```python
from build123d import *

# Parameters (mm, degrees)
SKETCH_1_W           = 185
SKETCH_1_H           = 55
EXTRUDE_1_DEPTH      = 25
SHELL_1_T            = -2
SKETCH_8_R           = 2.15
EXTRUDE_3_DEPTH      = 4
SKETCH_2_W           = 10
SKETCH_2_H           = 4
SKETCH_2_W_2         = 5
SKETCH_2_H_2         = 5
SKETCH_2_R           = 1.4
SKETCH_2_W_3         = 170
EXTRUDE_4_DEPTH      = 6
SKETCH_2_6_R         = 2.8
SKETCH_2_6_R_2       = 1.4
EXTRUDE_6_DEPTH      = 23
SKETCH_9_W           = 30
SKETCH_9_H           = 11
CUT_EXTRUDE_7_DEPTH  = 5
SKETCH_10_W          = 177
SKETCH_10_H          = 7.5
CUT_EXTRUDE_8_DEPTH  = 5
SKETCH_11_W          = 21.2
SKETCH_11_H          = 7.5
CUT_EXTRUDE_9_DEPTH  = 5
SKETCH_12_W          = 174
SKETCH_12_H          = 7.5
CUT_EXTRUDE_10_DEPTH = 5


with BuildPart() as part:
    # Sketch 1 → Extrude 1 (new body)
    with BuildSketch(Plane(origin=(0, 0, 0), x_dir=(1, 0, 0), z_dir=(0, 1, 0))):
        Rectangle(SKETCH_1_W, SKETCH_1_H)
    extrude(amount=EXTRUDE_1_DEPTH)

    # Shell 1
    shell_1_openings = [part.faces().sort_by_distance(p)[0] for p in [
        (0, 25, 0),
    ]]
    offset(amount=SHELL_1_T, openings=shell_1_openings, kind=Kind.INTERSECTION)

    # Sketch 8 → Extrude 3 (add)
    with BuildSketch(Plane.XZ):
        with BuildLine():
            Line((-97.5, 5), (-96, 5))
            Line((-96, 5), (-96, 27.5))
            Line((-96, 27.5), (-92.5, 27.5))
            Line((-92.5, 27.5), (-92.5, -27.5))
            Line((-92.5, -27.5), (-96, -27.5))
            Line((-96, -27.5), (-96, -5))
            Line((-96, -5), (-97.5, -5))
            ThreePointArc((-97.5, -5), (-102.5, 0), (-97.5, 5))
        make_face()
        with Locations((-97.5, 0)):
            Circle(SKETCH_8_R, mode=Mode.SUBTRACT)
        with BuildLine():
            Line((97.5, -5), (96, -5))
            Line((96, -5), (96, -27.5))
            Line((96, -27.5), (92.5, -27.5))
            Line((92.5, -27.5), (92.5, -5))
            Line((92.5, -5), (92.5, 5))
            Line((92.5, 5), (92.5, 27.5))
            Line((92.5, 27.5), (96, 27.5))
            Line((96, 27.5), (96, 5))
            Line((96, 5), (97.5, 5))
            ThreePointArc((97.5, 5), (102.5, 0), (97.5, -5))
        make_face()
        with Locations((97.5, 0)):
            Circle(SKETCH_8_R, mode=Mode.SUBTRACT)
    extrude(amount=-EXTRUDE_3_DEPTH)

    # Sketch 2 → Extrude 4 (add)
    with BuildSketch(Plane(origin=(0, 2, 0), x_dir=(1, 0, 0), z_dir=(0, 1, 0))):
        with Locations((-85.5, 23.4)):
            Rectangle(SKETCH_2_W, SKETCH_2_H)
        with Locations((-74.6, 12.65)):
            Rectangle(SKETCH_2_W_2, SKETCH_2_H_2)
        with Locations((-74.6, 12.65)):
            Circle(SKETCH_2_R, mode=Mode.SUBTRACT)
        with Locations((74.6, -12.65)):
            Rectangle(SKETCH_2_W_2, SKETCH_2_H_2)
        with Locations((74.6, -12.65)):
            Circle(SKETCH_2_R, mode=Mode.SUBTRACT)
        with Locations((74.6, 12.65)):
            Rectangle(SKETCH_2_W_2, SKETCH_2_H_2)
        with Locations((74.6, 12.65)):
            Circle(SKETCH_2_R, mode=Mode.SUBTRACT)
        with Locations((0, -12.65)):
            Rectangle(SKETCH_2_W_2, SKETCH_2_H_2)
        with Locations((0, -12.65)):
            Circle(SKETCH_2_R, mode=Mode.SUBTRACT)
        with Locations((0, 12.65)):
            Rectangle(SKETCH_2_W_2, SKETCH_2_H_2)
        with Locations((0, 12.65)):
            Circle(SKETCH_2_R, mode=Mode.SUBTRACT)
        with Locations((-0.5, -23.002466961)):
            Rectangle(SKETCH_2_W_3, SKETCH_2_H)
    extrude(amount=EXTRUDE_4_DEPTH)

    # Sketch 2_6 → Extrude 6 (add)
    with BuildSketch(Plane(origin=(0, 2, 0), x_dir=(1, 0, 0), z_dir=(0, 1, 0))):
        Circle(SKETCH_2_6_R)
        Circle(SKETCH_2_6_R_2, mode=Mode.SUBTRACT)
    extrude(amount=EXTRUDE_6_DEPTH)

    # Sketch 9 → Cut-Extrude 7 (cut)
    with BuildSketch(Plane(origin=(92.5, 0, 0), x_dir=(0, 0, -1), z_dir=(1, 0, 0))):
        with Locations((0.5, 11.9)):
            Rectangle(SKETCH_9_W, SKETCH_9_H)
    extrude(amount=-CUT_EXTRUDE_7_DEPTH, mode=Mode.SUBTRACT)

    # Sketch 10 → Cut-Extrude 8 (cut)
    with BuildSketch(Plane.XY.offset(27.5)):
        with Locations((0.2, 12.65)):
            Rectangle(SKETCH_10_W, SKETCH_10_H)
    extrude(amount=-CUT_EXTRUDE_8_DEPTH, mode=Mode.SUBTRACT)

    # Sketch 11 → Cut-Extrude 9 (cut)
    with BuildSketch(Plane.ZY.offset(92.5)):
        with Locations((-4.9, 12.65)):
            Rectangle(SKETCH_11_W, SKETCH_11_H)
    extrude(amount=-CUT_EXTRUDE_9_DEPTH, mode=Mode.SUBTRACT)

    # Sketch 12 → Cut-Extrude 10 (cut)
    with BuildSketch(Plane(origin=(0, 0, -27.5), x_dir=(-1, 0, 0), z_dir=(0, 0, -1))):
        with Locations((-0.5, 12.65)):
            Rectangle(SKETCH_12_W, SKETCH_12_H)
    extrude(amount=-CUT_EXTRUDE_10_DEPTH, mode=Mode.SUBTRACT)


solid = part.part
```
Here's how the part is built. I have some questions about the finished solid (model axes, mm). A direction names the side the tool comes from. Round coordinates to 2 decimals unless told otherwise and drop trailing zeros. Loops run counter-clockwise (first coordinate to the right, second up) from the corner with the lowest first, then second, coordinate; pieces in that order, holes last.
1. Will these pins go through, and if not, where does the flat tip stop? pin 1 (1 mm diameter, centred on y = 4, z = 6.5, fed in from -X); pin 2 (1 mm diameter, centred on y = 13, z = -26.5, fed in from +X); pin 3 (0.8 mm diameter, centred on x = 0.5, z = 12.5, fed in from +Y); pin 4 (5 mm diameter, centred on x = 68.5, y = 13.5, fed in from +Z).
Answers:
pin 1: stops at x = -96
pin 2: stops at x = 92.5
pin 3: stops at y = 2
pin 4: passes through
2. Thinking about a two-plate mould opening in Z: for faces 6 (the face through (1.2, 25, 1.2)), 7 (the face through (-2, 5, 21.002)), which applies, released by +Z, released by -Z, zero draft, split by the parting line, or undercut?
Answers:
face 6: zero draft
face 7: undercut
3. Suppose I cut it at B-B, the plane z = -8. Please give me the cut outline in (x, y).
Answers:
outline: (-96, 0) - (96, 0) - (96, 4) - (92.5, 4) - (92.5, 6.4) - (90.5, 6.4) - (90.5, 2) - (-90.5, 2) - (-90.5, 8.9) - (-92.5, 8.9) - (-92.5, 4) - (-96, 4) - close; (-92.5, 16.4) - (-90.5, 16.4) - (-90.5, 25) - (-92.5, 25) - close; (90.5, 17.4) - (92.5, 17.4) - (92.5, 25) - (90.5, 25) - close
4. For faces 1 (the face through (75, 5, -10.15)), 2 (the face through (92.5, 19, 0)), 3 (the face through (96, 2, -16)), 4 (the face through (-96, 2, 16)), 5 (the face through (-96, 2, -16)), which set-ups out of +Z, -Z, +X, -X, +Y, -Y let a thin tool reach every point of the face, with its end or its side?
Answers:
face 1: +Y
face 2: +Z, -Z, +X, +Y
face 3: -Z, +X, +Y, -Y
face 4: +Z, -X, +Y, -Y
face 5: -Z, -X, +Y, -Y
5. Suppose I cut it at C-C, the plane x = -38. Please give me the cut outline in (y, z).
Answers:
outline: (0, -27.5) - (8.9, -27.5) - (8.9, -25.5) - (2, -25.5) - (2, 21) - (8, 21) - (8, 25) - (2, 25) - (2, 25.5) - (8.9, 25.5) - (8.9, 27.5) - (0, 27.5) - close; (16.4, -27.5) - (25, -27.5) - (25, -25.5) - (16.4, -25.5) - close; (16.4, 25.5) - (25, 25.5) - (25, 27.5) - (16.4, 27.5) - close
6. Suppose I cut it at A-A, the plane y = 14. Please give me the cut outline in (x, z), and give its area (3 significant figures).
Answers:
outline: (-92.5, -27.5) - (-86.5, -27.5) - (-86.5, -25.5) - (-90.5, -25.5) - (-90.5, -15.5) - (-92.5, -15.5) - close; (-92.5, 5.7) - (-90.5, 5.7) - (-90.5, 25.5) - (-88.3, 25.5) - (-88.3, 27.5) - (-92.5, 27.5) - close; circle Ø5.6 at (0, 0); (87.5, -27.5) - (92.5, -27.5) - (92.5, -15.5) - (90.5, -15.5) - (90.5, -25.5) - (87.5, -25.5) - close; (88.7, 25.5) - (90.5, 25.5) - (90.5, 14.5) - (92.5, 14.5) - (92.5, 27.5) - (88.7, 27.5) - close; hole circle Ø2.8 at (0, 0)
area: 158 mm2
7. If I drill on probe 1 along X at (y, z) = (3.7, 12.65); probe 2 along Z at (x, y) = (35.5, 3.75); probe 3 along X at (y, z) = (19.5, 10), over which ranges is the centre line in solid material (lowest first)?
Answers:
probe 1: x = -96 to -90.5, -2.5 to -1.4, 1.4 to 2.5, 72.1 to 73.2, 76 to 77.1, 90.5 to 96
probe 2: z = -27.5 to -25.5, 21 to 25, 25.5 to 27.5
probe 3: x = -92.5 to -90.5, 90.5 to 92.5
